from build123d import *

# Parameters (mm, degrees)
CUT_EXTRUDE1_REACH = 67.609
SKETCH2_R          = 1.5875
CUT_EXTRUDE2_DEPTH = 2.8575
CIRPATTERN1_COUNT  = 6
CUT_EXTRUDE3_REACH = 67.609
SKETCH4_R          = 3


with BuildPart() as part:
    # Sketch1 → Revolve1 (revolve)
    with BuildSketch(Plane.XY, mode=Mode.PRIVATE) as revolve1_sk:
        Polygon((0, 0), (0, 40.5), (35, 40.5), (35, 37.5), (3, 37.5), (3, 0), align=None)
    revolve(revolve1_sk.sketch.rotate(Axis((0, 0, 0), (1, 0, 0)), 90), axis=Axis((0, 0, 0), (1, 0, 0)))

    # Sketch2 → Cut-Extrude1 (cut, up to next)
    with BuildSketch(Plane(origin=(3, 0, 0), x_dir=(0, 0, -1), z_dir=(1, 0, 0)), mode=Mode.PRIVATE) as cut_extrude1_sk1:
        with Locations((-31, 0)):
            Circle(SKETCH2_R)
    cut_extrude1_tool1 = extrude(cut_extrude1_sk1.sketch, amount=-CUT_EXTRUDE1_REACH, mode=Mode.PRIVATE) & part.part
    # Sketch2 → Cut-Extrude1 (cut, up to next)
    with BuildSketch(Plane(origin=(3, 0, 0), x_dir=(0, 0, -1), z_dir=(1, 0, 0)), mode=Mode.PRIVATE) as cut_extrude1_sk2:
        with Locations((-15.5, 26.846787517)):
            Circle(SKETCH2_R)
    cut_extrude1_tool2 = extrude(cut_extrude1_sk2.sketch, amount=-CUT_EXTRUDE1_REACH, mode=Mode.PRIVATE) & part.part
    # Sketch2 → Cut-Extrude1 (cut, up to next)
    with BuildSketch(Plane(origin=(3, 0, 0), x_dir=(0, 0, -1), z_dir=(1, 0, 0)), mode=Mode.PRIVATE) as cut_extrude1_sk3:
        with Locations((15.5, 26.846787517)):
            Circle(SKETCH2_R)
    cut_extrude1_tool3 = extrude(cut_extrude1_sk3.sketch, amount=-CUT_EXTRUDE1_REACH, mode=Mode.PRIVATE) & part.part
    # Sketch2 → Cut-Extrude1 (cut, up to next)
    with BuildSketch(Plane(origin=(3, 0, 0), x_dir=(0, 0, -1), z_dir=(1, 0, 0)), mode=Mode.PRIVATE) as cut_extrude1_sk4:
        with Locations((31, 0)):
            Circle(SKETCH2_R)
    cut_extrude1_tool4 = extrude(cut_extrude1_sk4.sketch, amount=-CUT_EXTRUDE1_REACH, mode=Mode.PRIVATE) & part.part
    # Sketch2 → Cut-Extrude1 (cut, up to next)
    with BuildSketch(Plane(origin=(3, 0, 0), x_dir=(0, 0, -1), z_dir=(1, 0, 0)), mode=Mode.PRIVATE) as cut_extrude1_sk5:
        with Locations((15.5, -26.846787517)):
            Circle(SKETCH2_R)
    cut_extrude1_tool5 = extrude(cut_extrude1_sk5.sketch, amount=-CUT_EXTRUDE1_REACH, mode=Mode.PRIVATE) & part.part
    # Sketch2 → Cut-Extrude1 (cut, up to next)
    with BuildSketch(Plane(origin=(3, 0, 0), x_dir=(0, 0, -1), z_dir=(1, 0, 0)), mode=Mode.PRIVATE) as cut_extrude1_sk6:
        with Locations((-15.5, -26.846787517)):
            Circle(SKETCH2_R)
    cut_extrude1_tool6 = extrude(cut_extrude1_sk6.sketch, amount=-CUT_EXTRUDE1_REACH, mode=Mode.PRIVATE) & part.part
    add(cut_extrude1_tool1.solids().sort_by_distance((3, 0, 31))[0], mode=Mode.SUBTRACT)
    add(cut_extrude1_tool2.solids().sort_by_distance((3, 26.846788, 15.5))[0], mode=Mode.SUBTRACT)
    add(cut_extrude1_tool3.solids().sort_by_distance((3, 26.846788, -15.5))[0], mode=Mode.SUBTRACT)
    add(cut_extrude1_tool4.solids().sort_by_distance((3, 0, -31))[0], mode=Mode.SUBTRACT)
    add(cut_extrude1_tool5.solids().sort_by_distance((3, -26.846788, -15.5))[0], mode=Mode.SUBTRACT)
    add(cut_extrude1_tool6.solids().sort_by_distance((3, -26.846788, 15.5))[0], mode=Mode.SUBTRACT)

    # Sketch3 → Cut-Extrude2 (cut)
    with BuildSketch(Plane(origin=(3, 0, 0), x_dir=(0, 0, -1), z_dir=(1, 0, 0))):
        Polygon((18.55, 25.085869196), (18.55, 28.607705838), (15.5, 30.368624159), (12.45, 28.607705838), (12.45, 25.085869196), (15.5, 23.324950875), align=None)
    cut_extrude2 = extrude(amount=-CUT_EXTRUDE2_DEPTH, mode=Mode.SUBTRACT)

    # CirPattern1: Cut-Extrude2 ×6 about axis
    cirpattern1_axis = Axis((0, 0, 0), (1, 0, 0))
    for i in range(1, CIRPATTERN1_COUNT):
        add(cut_extrude2.rotate(cirpattern1_axis, i * 360 / CIRPATTERN1_COUNT), mode=Mode.SUBTRACT)

    # Sketch4 → Cut-Extrude3 (cut, up to next)
    with BuildSketch(Plane(origin=(3, 0, 0), x_dir=(0, 0, -1), z_dir=(1, 0, 0)), mode=Mode.PRIVATE) as cut_extrude3_sk1:
        Circle(SKETCH4_R)
    cut_extrude3_tool1 = extrude(cut_extrude3_sk1.sketch, amount=-CUT_EXTRUDE3_REACH, mode=Mode.PRIVATE) & part.part
    add(cut_extrude3_tool1.solids().sort_by_distance((3, 0, 0))[0], mode=Mode.SUBTRACT)


solid = part.part
Build history of the part. All positions in model axes, mm. Coordinates: 2 decimals unless noted, no trailing zeros. Order: outer loops, then holes, each group sorted by start corner. A loop starts at its lowest first (then second) coordinate and runs counter-clockwise, first axis right, second up. Notation, with made-up numbers: (80, 45.25) - (111, 45.25) arc R26 ccw to (111, 80.25) - close; hole circle Ø2 at (71, -32). An arc over 180 degrees is marked (long way). Put each result on its own line as item: value.
1. Probe line 1 along Y through (x, z) = (0.1, 15.5); line 2 along X through (y, z) = (-4, 12); line 3 along Y through (x, z) = (20, 8.5). List the from-to ranges inside material, lowest first. Write a range as [from, to].
Answer sheet:
line 1: y = [-37.42, -28.43], [-25.26, 25.26], [28.43, 37.42]
line 2: x = [0, 3]
line 3: y = [-39.6, -36.52], [36.52, 39.6]
2. Drop flat-ended pins along their axis: P1, Ø5, axis at y = 0, z = -31, coming from the +X side; P2, Ø2.5, axis at x = 2, y = 27, coming from the +Z side; P3, Ø8, axis at x = 21, y = 29.5, coming from the +Z side. Give the stop position or say it passes through.
Answer sheet:
P1: stops at x = 0.14
P2: stops at z = 31.26
P3: stops at z = 31.46
3. Saw through at C-C (x = 10.5). Write the cut outline in (y, z), and give its area (3 significant figures).
Answer sheet:
outline: circle Ø81 at (0, 0); hole circle Ø75 at (0, 0)
area: 735 mm^2
4. Saw through at A-A (y = 0). Write the cut outline in (x, z).
Answer sheet:
outline: (0, -40.5) - (35, -40.5) - (35, -37.5) - (3, -37.5) - (3, -34.05) - (0.14, -34.05) - (0.14, -32.59) - (0, -32.59) - close; (0, -29.41) - (0.14, -29.41) - (0.14, -27.95) - (3, -27.95) - (3, -3) - (0, -3) - close; (0, 3) - (3, 3) - (3, 27.95) - (0.14, 27.95) - (0.14, 29.41) - (0, 29.41) - close; (0, 32.59) - (0.14, 32.59) - (0.14, 34.05) - (3, 34.05) - (3, 37.5) - (35, 37.5) - (35, 40.5) - (0, 40.5) - close
5. Saw through at D-D (y = -21.5). Write the cut outline in (x, z).
Answer sheet:
outline: (0, -34.32) - (35, -34.32) - (35, -30.72) - (3, -30.72) - (3, 30.72) - (35, 30.72) - (35, 34.32) - (0, 34.32) - close
6. Saw through at B-B (z = 0). Write the cut outline in (x, y), and give its area (3 significant figures).
Answer sheet:
outline: (0, -40.5) - (35, -40.5) - (35, -37.5) - (3, -37.5) - (3, -3) - (0, -3) - close; (0, 3) - (3, 3) - (3, 37.5) - (35, 37.5) - (35, 40.5) - (0, 40.5) - close
area: 417 mm^2
